from build123d import *

# Parameters (mm, degrees)
SKETCH1_W             = 82.68
SKETCH1_H             = 80.24
BOSS_EXTRUDE1_DEPTH   = 19
SKETCH2_W             = 79.68
SKETCH2_H             = 77.24
CUT_EXTRUDE1_DEPTH    = 18
CUT_EXTRUDE2_DEPTH    = 117.770886783
FILLET1_R             = 3
F_2_0MM_DOWEL_HOLE1_D = 2
RIB1_REACH            = 117.739
SKETCH5_WALLS_W       = 2.46
SKETCH5_WALLS_H       = 310.717342304


with BuildPart() as part:
    # Sketch1 → Boss-Extrude1 (new body)
    with BuildSketch(Plane(origin=(0, 0, 0), x_dir=(1, 0, 0), z_dir=(0, 1, 0))):
        with Locations((41.34, 40.12)):
            Rectangle(SKETCH1_W, SKETCH1_H)
    extrude(amount=BOSS_EXTRUDE1_DEPTH)

    # Sketch2 → Cut-Extrude1 (cut)
    with BuildSketch(Plane(origin=(0, 19, 0), x_dir=(1, 0, 0), z_dir=(0, 1, 0))):
        with Locations((41.34, 40.12)):
            Rectangle(SKETCH2_W, SKETCH2_H)
    extrude(amount=-CUT_EXTRUDE1_DEPTH, mode=Mode.SUBTRACT)

    # Sketch3 → Cut-Extrude2 (cut, through all)
    with BuildSketch(Plane(origin=(82.68, 0, 0), x_dir=(0, 0, -1), z_dir=(1, 0, 0))):
        with BuildLine():
            Line((27.37, 7), (52.87, 7))
            Line((52.87, 7), (52.87, 10))
            ThreePointArc((52.87, 10), (53.162893219, 10.707106781), (53.87, 11))
            Line((53.87, 11), (62.455786438, 11))
            ThreePointArc((62.455786438, 11), (62.83846987, 11.076120467), (63.162893219, 11.292893219))
            Line((63.162893219, 11.292893219), (66.819747468, 14.949747468))
            ThreePointArc((66.819747468, 14.949747468), (67.144170817, 15.16652022), (67.526854249, 15.242640687))
            Line((67.526854249, 15.242640687), (78.74, 15.242640687))
            Line((78.74, 15.242640687), (78.74, 19))
            Line((78.74, 19), (1.5, 19))
            Line((1.5, 19), (1.5, 15.242640687))
            Line((1.5, 15.242640687), (12.713145751, 15.242640687))
            ThreePointArc((12.713145751, 15.242640687), (13.095829183, 15.16652022), (13.420252532, 14.949747468))
            Line((13.420252532, 14.949747468), (17.077106781, 11.292893219))
            ThreePointArc((17.077106781, 11.292893219), (17.40153013, 11.076120467), (17.784213562, 11))
            Line((17.784213562, 11), (26.37, 11))
            ThreePointArc((26.37, 11), (27.077106781, 10.707106781), (27.37, 10))
            Line((27.37, 10), (27.37, 7))
        make_face()
    extrude(amount=-CUT_EXTRUDE2_DEPTH, mode=Mode.SUBTRACT)

    # Fillet1
    fillet1_edges = [part.edges().sort_by_distance(p)[0] for p in [
        (81.18, 1, -40.12),
        (1.5, 1, -40.12),
    ]]
    fillet(fillet1_edges, radius=FILLET1_R)

    # Ø2.0mm Dowel Hole1 (through all)
    with Locations(Plane(origin=(0, 0, 0), x_dir=(-1, 0, 0), z_dir=(0, -1, 0))):
        with Locations((-6.765, 57.42), (-17.115, 57.42), (-26.365, 57.42), (-36.715, 57.42), (-45.965, 57.42), (-56.315, 57.42), (-65.565, 57.42), (-75.915, 57.42), (-75.915, 22.82), (-65.565, 22.82), (-56.315, 22.82), (-45.965, 22.82), (-36.715, 22.82), (-26.365, 22.82), (-17.115, 22.82), (-6.765, 22.82)):
            Hole(F_2_0MM_DOWEL_HOLE1_D / 2)

    # Sketch5 walls → Rib1 (add, up to next)
    with BuildSketch(Plane(origin=(0, 11, 0), x_dir=(1, 0, 0), z_dir=(0, 1, 0)), mode=Mode.PRIVATE) as rib1_sk1:
        with Locations((20.94, 40.12)):
            Rectangle(SKETCH5_WALLS_W, SKETCH5_WALLS_H)
    rib1_tool1 = extrude(rib1_sk1.sketch, amount=-RIB1_REACH, mode=Mode.PRIVATE) - part.part
    # Sketch5 walls → Rib1 (add, up to next)
    with BuildSketch(Plane(origin=(0, 11, 0), x_dir=(1, 0, 0), z_dir=(0, 1, 0)), mode=Mode.PRIVATE) as rib1_sk2:
        with Locations((41.34, 40.12)):
            Rectangle(SKETCH5_WALLS_W, SKETCH5_WALLS_H)
    rib1_tool2 = extrude(rib1_sk2.sketch, amount=-RIB1_REACH, mode=Mode.PRIVATE) - part.part
    # Sketch5 walls → Rib1 (add, up to next)
    with BuildSketch(Plane(origin=(0, 11, 0), x_dir=(1, 0, 0), z_dir=(0, 1, 0)), mode=Mode.PRIVATE) as rib1_sk3:
        with Locations((61.74, 40.12)):
            Rectangle(SKETCH5_WALLS_W, SKETCH5_WALLS_H)
    rib1_tool3 = extrude(rib1_sk3.sketch, amount=-RIB1_REACH, mode=Mode.PRIVATE) - part.part
    add(rib1_tool1.solids().sort_by_distance((20.94, 11, -40.12))[0])
    add(rib1_tool2.solids().sort_by_distance((41.34, 11, -40.12))[0])
    add(rib1_tool3.solids().sort_by_distance((61.74, 11, -40.12))[0])


solid = part.part
Could you check a few things on this model? Use its own coordinates, in mm. A direction names the side the tool comes from. Coordinates: 2 decimals unless noted, no trailing zeros. Loops run counter-clockwise (first coordinate to the right, second up) from the corner with the lowest first, then second, coordinate; pieces in that order, holes last.
1. We'd pull the mould along Z, two halves only. Please class faces 4 (the face through (31, 1, -41)), 5 (the face through (41, 0, -41)): released by +Z, released by -Z, zero draft, split by the parting line, or undercut.
2. Imagine slicing it at B-B (y = 5.75). Please give me the cut outline in (x, z).
3. Imagine slicing it at C-C (z = -36.5). Please give me the cut outline in (x, y).
4. Imagine slicing it at A-A (y = 12.25). Please give me the cut outline in (x, z).
5. For P1, Ø1.6, axis at x = 6.765, z = -22.82, coming from the +Y side; P2, Ø1, axis at y = 4, z = -64.5, coming from the -X side; P3, Ø1.2, axis at x = 82, z = -5.5, coming from the +Y side; P4, Ø1.6, axis at x = 82, z = -42, coming from the +Y side, each with a flat end and sliding along its axis, tell me the tip position at first contact or that it passes through.
6. For faces 1 (the face through (81.94, 13.15, -15.22)), 2 (the face through (42, 12, -78.74)), 3 (the face through (35.716, 0.507, -22.864)), which set-ups out of +Z, -Z, +X, -X, +Y, -Y let a thin tool reach every point of the face, with its end or its side?
7. I need wall thicknesses on L1, parallel to X at y = 4.5, z = -58; L2, parallel to Z at x = 69, y = 2.5; L3, parallel to Y at x = 23.5, z = -22.5. Which ranges of each line are inside material? Lowest first, please.
8. Imagine slicing it at D-D (x = 32). Please give me the cut outline in (y, z), and give its area (3 significant figures).
Computed values:
1. face 4: undercut
1. face 5: zero draft
2. outline: (0, -80.24) - (82.68, -80.24) - (82.68, 0) - (0, 0) - close; hole (1.5, -78.74) - (19.71, -78.74) - (19.71, -1.5) - (1.5, -1.5) - close; hole (22.17, -78.74) - (40.11, -78.74) - (40.11, -1.5) - (22.17, -1.5) - close; hole (42.57, -78.74) - (60.51, -78.74) - (60.51, -1.5) - (42.57, -1.5) - close; hole (62.97, -78.74) - (81.18, -78.74) - (81.18, -1.5) - (62.97, -1.5) - close
3. outline: (0, 0) - (82.68, 0) - (82.68, 7) - (81.18, 7) - (81.18, 4) arc R3 cw to (78.18, 1) - (62.97, 1) - (62.97, 11) - (60.51, 11) - (60.51, 1) - (42.57, 1) - (42.57, 11) - (40.11, 11) - (40.11, 1) - (22.17, 1) - (22.17, 11) - (19.71, 11) - (19.71, 1) - (4.5, 1) arc R3 cw to (1.5, 4) - (1.5, 7) - (0, 7) - close
4. outline: (0, -80.24) - (82.68, -80.24) - (82.68, -64.12) - (81.18, -64.12) - (81.18, -78.74) - (1.5, -78.74) - (1.5, -64.12) - (0, -64.12) - close; (0, -16.12) - (1.5, -16.12) - (1.5, -1.5) - (81.18, -1.5) - (81.18, -16.12) - (82.68, -16.12) - (82.68, 0) - (0, 0) - close
5. P1: passes through
5. P2: stops at x = 0
5. P3: stops at y = 15.24
5. P4: stops at y = 7
6. face 1: +X, -X, +Y
6. face 2: +Y
6. face 3: +Y, -Y
7. L1: x = 0 to 1.5, 19.71 to 22.17, 40.11 to 42.57, 60.51 to 62.97, 81.18 to 82.68
7. L2: z = -80.24 to -78.74, -1.5 to 0
7. L3: y = 0 to 1
8. outline: (0, -80.24) - (19, -80.24) - (19, -78.74) - (1, -78.74) - (1, -1.5) - (19, -1.5) - (19, 0) - (0, 0) - close
8. area: 134 mm2
